Geometry: final body of the model. Coordinates: model frame, mm. Give positions to 0.01 mm unless a question says otherwise; leave off trailing zeros. Write each loop counter-clockwise with the first axis right and the second up, starting at its lowest first coordinate (ties: lowest second). Pieces come first, ordered by that corner, then holes.
Q1. Section B-B (y = -46.15). State how many separate pieces and enclosed holes the cut face has, plus the area to 3 significant figures.
Q2. Line query: line 1 (Z direction, x = 32.5, y = -46.1). Output: solid intervals per line, ascending.
Q3. Pin query (flat end, axial travel): pin 1 Ø6 at (x, z) = (9, 25.5) entering from +Y. Return the tip coordinate at first contact, or that it passes through.
Q4. Section A-A (x = 39). Return the cut outline in (y, z), plus the area to 3 significant figures.
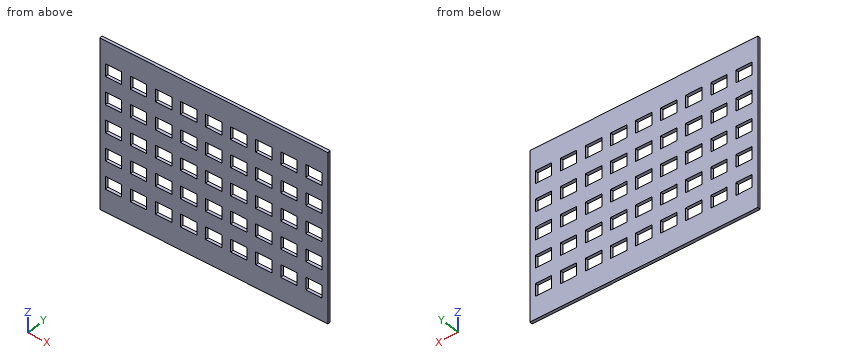
from build123d import *

# Parameters (mm, degrees)
BOX007_W         = 6.5
BOX007_H         = 5
BOX007_DEPTH     = 5
ARRAY001_X_COUNT = 9
ARRAY001_X_PITCH = 10
ARRAY001_Z_COUNT = 5
ARRAY001_Z_PITCH = 11
BOX006_W         = 91
BOX006_H         = 67
BOX006_DEPTH     = 1.2


with BuildPart() as array001:
    # Box007 → Box007 (new body)
    with BuildSketch(Plane(origin=(-43, -3, 11), x_dir=(1, 0, 0), z_dir=(0, 0, 1))):
        with Locations((3.25, 2.5)):
            Rectangle(BOX007_W, BOX007_H)
    extrude(amount=BOX007_DEPTH)

    # Array001 X: Array001 ×9


with BuildPart() as array001_1:
    add(array001.part)
    with Locations(*[(i * ARRAY001_X_PITCH, 0, 0) for i in range(1, ARRAY001_X_COUNT)]):
        add(array001.part)

    # Array001 Z: Array001 ×5


with BuildPart() as array001_2:
    add(array001_1.part)
    with Locations(*[(0, 0, i * ARRAY001_Z_PITCH) for i in range(1, ARRAY001_Z_COUNT)]):
        add(array001_1.part)


with BuildPart() as array001_3:
    # Array001 placement: moved
    add(array001_2.part.moved(Location((0.35, 0, -0.4))))


with BuildPart() as obj1:
    # Box006 → Box006 (new body)
    with BuildSketch(Plane(origin=(-44.9, 0, 1.6), x_dir=(1, 0, 0), z_dir=(0, -1, 0))):
        with Locations((45.5, 33.5)):
            Rectangle(BOX006_W, BOX006_H)
    extrude(amount=BOX006_DEPTH)

    # Cut003: cut Array001
    add(array001_3.part, mode=Mode.SUBTRACT)


with BuildPart() as obj1_1:
    # Cut003 placement: moved
    add(obj1.part.moved(Location((0, -45.2, 0))))


solid = obj1_1.part
Computed:
1. separate pieces: 1
1. enclosed holes: 45
1. area: 4,630 mm2
2. line 1: z = 1.6 to 10.6, 15.6 to 21.6, 26.6 to 32.6, 37.6 to 43.6, 48.6 to 54.6, 59.6 to 68.6
3. pin 1: stops at y = -45.2
4. outline: (-46.4, 1.6) - (-45.2, 1.6) - (-45.2, 10.6) - (-46.4, 10.6) - close; (-46.4, 15.6) - (-45.2, 15.6) - (-45.2, 21.6) - (-46.4, 21.6) - close; (-46.4, 26.6) - (-45.2, 26.6) - (-45.2, 32.6) - (-46.4, 32.6) - close; (-46.4, 37.6) - (-45.2, 37.6) - (-45.2, 43.6) - (-46.4, 43.6) - close; (-46.4, 48.6) - (-45.2, 48.6) - (-45.2, 54.6) - (-46.4, 54.6) - close; (-46.4, 59.6) - (-45.2, 59.6) - (-45.2, 68.6) - (-46.4, 68.6) - close
4. area: 50.4 mm2
